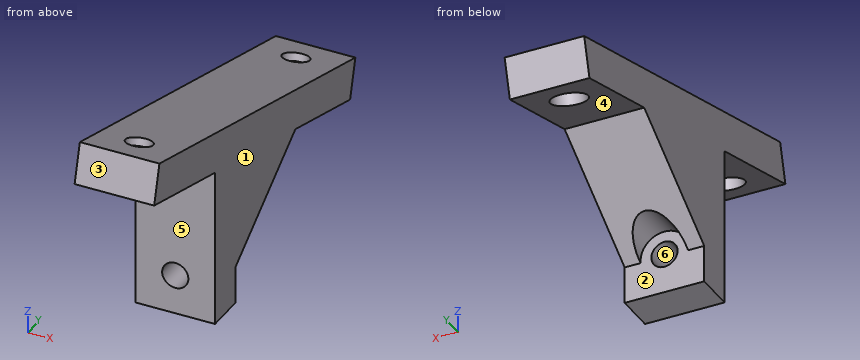
from build123d import *

# Parameters (mm, degrees)
EXTRUDE_2_DEPTH          = 10
SKETCH_3_R               = 1.65
CUT_EXTRUDE_2_DEPTH      = 10
CUT_EXTRUDE_3_DEPTH      = 10
CUT_EXTRUDE_3_DEPTH_BACK = 9
SKETCH_5_R               = 1.65
SKETCH_6_R               = 3
CUT_EXTRUDE_4_DEPTH      = 8
SKETCH_7_R               = 2.25
CUT_EXTRUDE_5_DEPTH      = 4


with BuildPart() as part:
    # 草图1 → 凸台-拉伸2 (new body)
    with BuildSketch(Plane(origin=(0, 0, 0), x_dir=(0, 0, -1), z_dir=(1, 0, 0))):
        Polygon((0, 0), (12.940952255, 48.296291314), (17.770581387, 47.002196089), (14.155128272, 33.509141372), (24.163916678, 18.705904774), (28.848867018, 18.705904774), (28.848867018, 13.705904774), (8.848867018, 13.705904774), (4.829629131, -1.294095226), align=None)
    extrude(amount=EXTRUDE_2_DEPTH)

    # 草图3 → 切除-拉伸2 (cut)
    with BuildSketch(Plane(origin=(0, -1.294095226, -4.829629131), x_dir=(-1, 0, 0), z_dir=(0, -0.2588190451025247, -0.9659258262890673))):
        with Locations(Location((-5, 45, 0), (0, 0, 90))):
            Circle(SKETCH_3_R)
        with Locations(Location((-5, 5, 0), (0, 0, 90))):
            Circle(SKETCH_3_R)
    extrude(amount=-CUT_EXTRUDE_2_DEPTH, mode=Mode.SUBTRACT)

    # 草图5 → 切除-拉伸3 (cut, two sides: drawn at the far end of the back side and taken through both)
    with BuildSketch(Plane(origin=(0, 18.705904774, 0), x_dir=(1, 0, 0), z_dir=(0, 1, 0)).offset(-CUT_EXTRUDE_3_DEPTH_BACK)):
        with Locations(Location((5, 23.848867018, 0), (0, 0, 90))):
            Circle(SKETCH_5_R)
    extrude(amount=CUT_EXTRUDE_3_DEPTH + CUT_EXTRUDE_3_DEPTH_BACK, mode=Mode.SUBTRACT)

    # 草图6 → 切除-拉伸4 (cut)
    with BuildSketch(Plane(origin=(0, 18.705904774, 0), x_dir=(1, 0, 0), z_dir=(0, 1, 0))):
        with Locations((5, 23.848867018)):
            Circle(SKETCH_6_R)
    extrude(amount=CUT_EXTRUDE_4_DEPTH, mode=Mode.SUBTRACT)

    # 草图7 → 切除-拉伸5 (cut)
    with BuildSketch(Plane(origin=(0, -1.294095226, -4.829629131), x_dir=(-1, 0, 0), z_dir=(0, -0.25881904510252446, -0.9659258262890674))):
        with Locations(Location((-5, 45, 0), (0, 0, 90))):
            Circle(SKETCH_7_R)
        with Locations(Location((-5, 5, 0), (0, 0, 90))):
            Circle(SKETCH_7_R)
    extrude(amount=-CUT_EXTRUDE_5_DEPTH, mode=Mode.SUBTRACT)


solid = part.part
Model file for the job. Use its own axes, mm. Face numbers are marked on the shaded views. A direction names the side the tool comes from. Round coordinates to 2 decimals unless told otherwise and drop trailing zeros. Order: outer loops, then holes, each group sorted by start corner. A loop starts at its lowest first (then second) coordinate and runs counter-clockwise, first axis right, second up.
(1) Band-saw the part on B-B (z = -22.75). List the corners of the cut face in (x, y).
(2) Band-saw the part on C-C (x = 0.75). List the corners of the cut face in (y, z), then the cut area to 3 significant figures.
(3) Band-saw the part on A-A (x = 5). Give the number of separate pieces and of enclosed holes in the cut face, then the cut area to 3 significant figures.
(4) Drill centre lines: line 1 (Y direction, x = 5.75, z = -26); line 2 (Y direction, x = 4, z = -1.25); line 3 (Z direction, x = 5, y = 20.2). Where is each one in solid material? Low to high.
(5) Pull direction X, two halves, no side cores. Call the marked faces 1, 2 and 3: released by +X, released by -X, zero draft, split by the parting line, or undercut.
(6) Pin check, flat tips, straight feed: pin 1 (4 mm diameter, centred on x = 5.5, z = -24, fed in from +Y); pin 2 (3 mm diameter, centred on y = 15, z = -7.5, fed in from -X); pin 3 (3 mm diameter, centred on x = 6.5, z = -21.5, fed in from -Y); pin 4 (4 mm diameter, centred on x = 1, y = 24.5, fed in from -Z). Stop position of each tip, or through.
(7) 3-axis set-ups, long thin cutter, end or side, ignore diameter. For the marked faces 4, 5 and 6: which of +Z, -Z, +X, -X, +Y, -Y reach the whole face in a straight line?
Verdict:
1. outline: (0, 13.71) - (3.77, 13.71) - (3.77, 18.71) - (2.21, 18.71) - (2.21, 20.8) - (0, 20.8) - close; (6.23, 13.71) - (10, 13.71) - (10, 20.8) - (7.79, 20.8) - (7.79, 18.71) - (6.23, 18.71) - close
2. outline: (-1.29, -4.83) - (13.71, -8.85) - (13.71, -28.85) - (18.71, -28.85) - (18.71, -24.16) - (33.51, -14.16) - (47, -17.77) - (48.3, -12.94) - (0, 0) - close
2. area: 450 mm2
3. separate pieces: 4
3. enclosed holes: 0
3. area: 383 mm2
4. line 1: y = 13.71 to 18.71
4. line 2: y = -0.33 to 3.48
4. line 3: z = -20.85 to -5.41
5. face 1: released by +X
5. face 2: undercut
5. face 3: zero draft
6. pin 1: stops at y = 18.71
6. pin 2: stops at x = 0
6. pin 3: stops at y = 13.71
6. pin 4: stops at z = -21.6
7. face 4: -Z, +X, -X
7. face 5: -Z, +X, -X, -Y
7. face 6: +Y, -Y
